```python
from build123d import *

# Parameters (mm, degrees)
SKETCH1_W           = 38.1
SKETCH1_H           = 25.4
BOSS_EXTRUDE1_DEPTH = 1.5875
SKETCH2_W           = 38.1
SKETCH2_H           = 28.575
BOSS_EXTRUDE2_DEPTH = 1.778
SKETCH3_W           = 38.1
SKETCH3_H           = 3.175
BOSS_EXTRUDE3_DEPTH = 25.4
SKETCH5_R           = 9.525
CUT_EXTRUDE1_DEPTH  = 51.973693058
CHAMFER1_SIZE       = 7.62
FILLET1_R           = 6.35
FILLET2_R           = 1.778


with BuildPart() as part:
    # Sketch1 → Boss-Extrude1 (new, symmetric)
    with BuildSketch(Plane.XY):
        Rectangle(SKETCH1_W, SKETCH1_H)
    extrude(amount=BOSS_EXTRUDE1_DEPTH, both=True)

    # Sketch2 → Boss-Extrude2 (add)
    with BuildSketch(Plane(origin=(0, 12.7, 0), x_dir=(1, 0, 0), z_dir=(0, 1, 0))):
        with Locations((0, 12.7)):
            Rectangle(SKETCH2_W, SKETCH2_H)
    extrude(amount=BOSS_EXTRUDE2_DEPTH)

    # Sketch3 → Boss-Extrude3 (add)
    with BuildSketch(Plane(origin=(0, 14.478, 0), x_dir=(1, 0, 0), z_dir=(0, 1, 0))):
        with Locations((0, 25.4)):
            Rectangle(SKETCH3_W, SKETCH3_H)
    extrude(amount=BOSS_EXTRUDE3_DEPTH)

    # Sketch5 → Cut-Extrude1 (cut, through all)
    with BuildSketch(Plane.XY.offset(-23.8125)):
        with Locations((0, 26.924)):
            Circle(SKETCH5_R)
    extrude(amount=-CUT_EXTRUDE1_DEPTH, mode=Mode.SUBTRACT)

    # Chamfer1
    chamfer1_edges = [part.edges().sort_by_distance(p)[0] for p in [
        (-19.05, 39.878, -25.4),
        (19.05, 39.878, -25.4),
    ]]
    chamfer(chamfer1_edges, length=CHAMFER1_SIZE)

    # Fillet1
    fillet1_edges = [part.edges().sort_by_distance(p)[0] for p in [
        (-19.05, 32.258, -25.4),
        (-11.43, 39.878, -25.4),
        (19.05, 32.258, -25.4),
        (11.43, 39.878, -25.4),
    ]]
    fillet(fillet1_edges, radius=FILLET1_R)

    # Fillet2
    fillet2_edges = [part.edges().sort_by_distance(p)[0] for p in [
        (0, 14.478, -23.8125),
    ]]
    fillet(fillet2_edges, radius=FILLET2_R)


solid = part.part
```
Verification items for the finished model (mm, model axes). A direction names the side the tool comes from. Coordinates: 2 decimals unless noted, no trailing zeros. Write each loop counter-clockwise with the first axis right and the second up, starting at its lowest first coordinate (ties: lowest second). Pieces come first, ordered by that corner, then holes. Notation, with made-up numbers: (62, -35.5) - (99, -35.5) arc R10 cw to (99, -31.5) - close; hole circle Ø4 at (34, 88). An arc over 180 degrees is marked (long way). One line per question, with ' | ' between items. Start each with the question number.
1. Section check D-D (z = -4.5). Enter the section's corners in (x, y), plus the area to 3 significant figures.
2. Section check B-B (y = 23). Enter the section's corners in (x, z).
3. Material ranges on line 1 along Y through (x, z) = (0, -25.85); line 2 along Z through (x, y) = (-16, -9); line 3 along Y through (x, z) = (-2, 0.25), recorded low to high.
4. Gauge pin test, flat ends, axial feed: P1, Ø20.5, axis at x = -4, y = -6.5, coming from the -Z side; P2, Ø7, axis at x = -3.5, z = -7, coming from the +Y side; P3, Ø10, axis at y = 30.5, z = -16, coming from the +X side. Record the tip position at first contact, or that the pin passes through.
5. Section check C-C (x = -12.5). Enter the section's corners in (y, z).
6. Access from +Z, -Z, +X, -X, +Y, -Y to the whole of each face (thin tool, end or side, straight path). Record for faces 4 (the flat face through (0, 0, -1.588)), 5 (the flat face through (0, 14.478, -10)), 6 (the flat face through (15.27, 36.04, -25.38)).
7. Section check A-A (x = 0). Enter the section's corners in (y, z), plus the area to 3 significant figures.
8. Draft check along X on faces 1 (the flat face through (0, 17, -26.987)), 2 (the cylindrical face through (-2.065, 17.626, -25.378)), 3 (the cylindrical face through (11.197, 39.408, -25.422)). Enter one of: released by +X, released by -X, zero draft, split by the parting line, or undercut.
Computed values:
1) outline: (-19.05, 12.7) - (19.05, 12.7) - (19.05, 14.48) - (-19.05, 14.48) - close | area: 67.7 mm²
2) outline: (-19.05, -26.99) - (-8.68, -26.99) - (-8.68, -23.81) - (-19.05, -23.81) - close; (8.68, -26.99) - (19.05, -26.99) - (19.05, -23.81) - (8.68, -23.81) - close
3) line 1: 12.7 to 17.4, 36.45 to 39.88 | line 2: -1.59 to 1.59 | line 3: -12.7 to 14.48
4) P1: z = -1.59 | P2: y = 14.48 | P3: through
5) outline: (-12.7, -1.59) - (12.7, -1.59) - (12.7, -26.99) - (38.69, -26.99) - (38.69, -23.81) - (16.26, -23.81) arc R1.78 cw to (14.48, -22.03) - (14.48, 1.59) - (-12.7, 1.59) - close
6) face 4: -Z, +X, -X, -Y | face 5: +Z, +X, -X, +Y | face 6: +Z, -Z, +X, +Y
7) outline: (-12.7, -1.59) - (12.7, -1.59) - (12.7, -26.99) - (17.4, -26.99) - (17.4, -23.81) - (16.26, -23.81) arc R1.78 cw to (14.48, -22.03) - (14.48, 1.59) - (-12.7, 1.59) - close; (36.45, -26.99) - (39.88, -26.99) - (39.88, -23.81) - (36.45, -23.81) - close | area: 152 mm²
8) face 1: zero draft | face 2: undercut | face 3: released by +X
